from build123d import *

# Parameters (mm, degrees)
SKETCH_W     = 280
SKETCH_H     = 180
PAD_DEPTH    = 44
SKETCH001_W  = 30
SKETCH001_H  = 54
PAD001_DEPTH = 10


with BuildPart() as pad:
    # Sketch → Pad (new body)
    with BuildSketch(Plane.XY):
        Rectangle(SKETCH_W, SKETCH_H)
    extrude(amount=PAD_DEPTH)


with BuildPart() as fusion:
    # Sketch001 → Pad001 (new body)
    with BuildSketch(Plane.XY):
        with Locations((155, -63)):
            Rectangle(SKETCH001_W, SKETCH001_H)
        with Locations((-155, -63)):
            Rectangle(SKETCH001_W, SKETCH001_H)
    extrude(amount=PAD001_DEPTH)

    # Fusion: union Pad
    add(pad.part)


solid = fusion.part
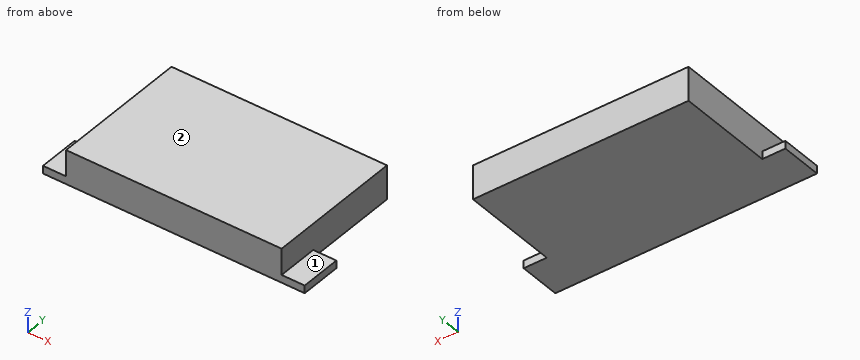
Geometry check sheet. Reference: the model listing, model coordinates, mm. Face numbers are marked on the shaded views. A direction names the side the tool comes from. Give positions to 0.01 mm unless a question says otherwise; leave off trailing zeros. Write each loop counter-clockwise with the first axis right and the second up, starting at its lowest first coordinate (ties: lowest second). Pieces come first, ordered by that corner, then holes. Notation, with made-up numbers: M 28.5,40 L 58.5,40 A13 cw 58.5,50 Z; hole C -21,44 d2. An arc over 180 degrees is marked long. Answer as CSV lines item,"result". Start each with the question number.
Q1. Section check B-B, the plane y = -66. Record the cut outline in (x, z), then the cut area to 3 significant figures.
Q2. Material ranges on L1, parallel to X at y = 17.5, z = 8; L2, parallel to Z at x = -145.5, y = -55, recorded low to high.
Q3. Section check D-D, the plane y = -12. Record the cut outline in (x, z).
Q4. Go/stop test with flat-tipped pins: pin 1 (15 mm diameter, centred on x = 156.5, y = -51.5, fed in from +Z); pin 2 (8 mm diameter, centred on x = -154.5, z = 4, fed in from +Y); pin 3 (4 mm diameter, centred on y = 47.5, z = 6, fed in from -X). Record where each tip stops, or that it passes through.
Q5. Section check A-A, the plane z = 6. Record the cut outline in (x, y), then the cut area to 3 significant figures.
Q6. Tool access check on the marked faces 1 and 2. Record the directions out of +Z, -Z, +X, -X, +Y, -Y that give a thin tool (end or side, any length) a straight path to the whole face; none if there is none.
Q7. Section check C-C, the plane x = 143.5. Record the cut outline in (y, z).
Geometry says:
1,outline,"M -170,0 L 170,0 L 170,10 L 140,10 L 140,44 L -140,44 L -140,10 L -170,10 Z"
1,area,"12,900 mm^2"
2,L1,"-140 to 140"
2,L2,"0 to 10"
3,outline,"M -140,0 L 140,0 L 140,44 L -140,44 Z"
4,pin 1,"z = 10"
4,pin 2,"y = -36"
4,pin 3,"x = -140"
5,outline,"M -170,-90 L 170,-90 L 170,-36 L 140,-36 L 140,90 L -140,90 L -140,-36 L -170,-36 Z"
5,area,"53,600 mm^2"
6,face 1,"+Z, +X, +Y, -Y"
6,face 2,"+Z, +X, -X, +Y, -Y"
7,outline,"M -90,0 L -36,0 L -36,10 L -90,10 Z"
